```python
from build123d import *

# Parameters (mm, degrees)
SKETCH1_W           = 148.5
SKETCH1_H           = 54.85
SKETCH1_R           = 1.5
BOSS_EXTRUDE1_DEPTH = 2.85
SKETCH2_W           = 21
SKETCH2_H           = 21
BOSS_EXTRUDE2_DEPTH = 13


with BuildPart() as part:
    # Sketch1 → Boss-Extrude1 (new body)
    # profile 1 of 2: a face of its own
    with BuildSketch(Plane(origin=(0, 0, 0), x_dir=(1, 0, 0), z_dir=(0, 1, 0))):
        with Locations((74.25, -27.425)):
            Rectangle(SKETCH1_W, SKETCH1_H)
        with Locations(Location((90.25, -5, 0), (0, 0, 270))):
            Circle(SKETCH1_R, mode=Mode.SUBTRACT)
        with Locations(Location((60.9, -5, 0), (0, 0, 270))):
            Circle(SKETCH1_R, mode=Mode.SUBTRACT)
        with Locations(Location((60.9, -49.85, 0), (0, 0, 270))):
            Circle(SKETCH1_R, mode=Mode.SUBTRACT)
        with Locations(Location((90.25, -49.85, 0), (0, 0, 270))):
            Circle(SKETCH1_R, mode=Mode.SUBTRACT)
    # profile 2 of 2: a face of its own
    with BuildSketch(Plane(origin=(0, 0, 0), x_dir=(1, 0, 0), z_dir=(0, 1, 0))):
        with BuildLine():
            Line((0, 0), (0, -54.85))
            ThreePointArc((0, -54.85), (-4.330823938, -27.425), (0, 0))
        make_face()
    extrude(amount=BOSS_EXTRUDE1_DEPTH)

    # Sketch2 → Boss-Extrude2 (add)
    with BuildSketch(Plane(origin=(0, 2.85, 0), x_dir=(1, 0, 0), z_dir=(0, 1, 0))):
        with Locations((74.75319094, -26.769521426)):
            Rectangle(SKETCH2_W, SKETCH2_H)
    extrude(amount=BOSS_EXTRUDE2_DEPTH)


solid = part.part
```
CAD build for the part. Positions are in the model's coordinates, mm. A direction names the side the tool comes from. Round coordinates to 2 decimals unless told otherwise and drop trailing zeros. Order: outer loops, then holes, each group sorted by start corner. A loop starts at its lowest first (then second) coordinate and runs counter-clockwise, first axis right, second up.
Item 1: Saw through at A-A on x = 90.25. Write the cut outline in (y, z), then the cut area to 3 significant figures.
Item 2: Saw through at B-B on z = 5. Write the cut outline in (x, y), then the cut area to 3 significant figures.
Item 3: Probe line 1 along Z through (x, y) = (90.25, 0.65); line 2 along X through (y, z) = (1.65, 49.85); line 3 along Y through (x, z) = (102, 17). List the from-to ranges inside material, lowest first.
Item 4: Pin check, flat tips, straight feed: pin 1 (4 mm diameter, centred on x = 67.5, z = 41.5, fed in from +Y); pin 2 (3.5 mm diameter, centred on x = 90.25, z = 5, fed in from -Y); pin 3 (6.5 mm diameter, centred on x = 76, y = 9.5, fed in from +Z); pin 4 (4 mm diameter, centred on y = 3.5, z = 25, fed in from -X). Stop position of each tip, or through.
Item 5: Saw through at C-C on x = 71. Write the cut outline in (y, z), then the cut area to 3 significant figures.
Item 6: Saw through at D-D on z = 30.5. Write the cut outline in (x, y), then the cut area to 3 significant figures.
Item 7: Tool access for faces 5 (the face through (64.253, 9, 27)), 6 (the face through (75, 9, 37.27)), 7 (the face through (85.253, 9, 27)), 8 (the face through (75, 9, 16.27)): list every direction of +Z, -Z, +X, -X, +Y, -Y with a clear straight run to the whole face (end or side of a thin tool).
Item 8: Mould opens along X. For faces 1 (the face through (-4.33, 1.41, 27.82)), 2 (the face through (148.5, 1, 28)), 3 (the face through (62.387, 1.405, 49.655)), 4 (the face through (73, 0, 27)) say: pulls with the +X half, pulls with the -X half, needs draft (parallel to the pull), parting line crosses it, or undercut.
Reported:
1. outline: (0, 0) - (2.85, 0) - (2.85, 3.5) - (0, 3.5) - close; (0, 6.5) - (2.85, 6.5) - (2.85, 48.35) - (0, 48.35) - close; (0, 51.35) - (2.85, 51.35) - (2.85, 54.85) - (0, 54.85) - close
1. area: 139 mm2
2. outline: (-1.46, 0) - (59.4, 0) - (59.4, 2.85) - (-1.46, 2.85) - close; (62.4, 0) - (88.75, 0) - (88.75, 2.85) - (62.4, 2.85) - close; (91.75, 0) - (148.5, 0) - (148.5, 2.85) - (91.75, 2.85) - close
2. area: 410 mm2
3. line 1: z = 0 to 3.5, 6.5 to 48.35, 51.35 to 54.85
3. line 2: x = -1.46 to 59.4, 62.4 to 88.75, 91.75 to 148.5
3. line 3: y = 0 to 2.85
4. pin 1: stops at y = 2.85
4. pin 2: stops at y = 0
4. pin 3: stops at z = 37.27
4. pin 4: stops at x = -4.33
5. outline: (0, 0) - (2.85, 0) - (2.85, 16.27) - (15.85, 16.27) - (15.85, 37.27) - (2.85, 37.27) - (2.85, 54.85) - (0, 54.85) - close
5. area: 429 mm2
6. outline: (-4.28, 0) - (148.5, 0) - (148.5, 2.85) - (85.25, 2.85) - (85.25, 15.85) - (64.25, 15.85) - (64.25, 2.85) - (-4.28, 2.85) - close
6. area: 708 mm2
7. face 5: +Z, -Z, -X, +Y
7. face 6: +Z, +X, -X, +Y
7. face 7: +Z, -Z, +X, +Y
7. face 8: -Z, +X, -X, +Y
8. face 1: pulls with the -X half
8. face 2: pulls with the +X half
8. face 3: undercut
8. face 4: needs draft
